Here's how the part is built. I have some questions about the finished solid (model axes, mm). Face numbers are marked on the shaded views. A direction names the side the tool comes from. Round coordinates to 2 decimals unless told otherwise and drop trailing zeros. Write each loop counter-clockwise with the first axis right and the second up, starting at its lowest first coordinate (ties: lowest second). Pieces come first, ordered by that corner, then holes. Notation, with made-up numbers: (33, 25) - (81, 25) arc R7 cw to (81, 37) - close; hole circle Ø11 at (6, 2.5). An arc over 180 degrees is marked (long way). One line per item, written item: value. Start each with the question number.
Item 1: Imagine slicing it at A-A, the plane y = 0. Please give me the cut outline in (x, z), then the cut area to 3 significant figures.
Item 2: If I drill on line 1 (Y direction, x = 20.75, z = -1.2); line 2 (Z direction, x = -2, y = -11.25); line 3 (X direction, y = 2.5, z = -10), over which ranges is the centre line in solid material (lowest first)?
Item 3: Imagine slicing it at B-B, the plane x = 20.75. Please give me the cut outline in (y, z), then the cut area to 3 significant figures.
Item 4: Imagine slicing it at D-D, the plane z = -9.5. Please give me the cut outline in (x, y).
Item 5: For P1, Ø3, axis at x = 21.5, z = -1.5, coming from the +Y side; P2, Ø6, axis at y = 5.5, z = -12.5, coming from the +X side; P3, Ø5, axis at x = 20.75, y = 0, coming from the -Z side; P4, Ø1.5, axis at x = -18.5, y = 9, coming from the -Z side, each with a flat end and sliding along its axis, tell me the tip position at first contact or that it passes through.
Item 6: Imagine slicing it at C-C, the plane x = 0. Please give me the cut outline in (y, z).
Item 7: For the marked faces 1 and 2, which set-ups out of +Z, -Z, +X, -X, +Y, -Y let a thin tool reach every point of the face, with its end or its side?
```python
from build123d import *

# Parameters (mm, degrees)
BOSS_EXTRUDE2_DEPTH = 2.6
SKETCH2_R           = 9
BOSS_EXTRUDE3_DEPTH = 16
REVOLVE1_ANGLE      = 180
SKETCH5_R           = 1.5
CUT_EXTRUDE1_DEPTH  = 16


with BuildPart() as part:
    # Sketch1 → Boss-Extrude2 (new body)
    with BuildSketch(Plane.XY):
        with BuildLine():
            Line((-26, -7.25), (-26, 7.25))
            Line((-26, 7.25), (-13.13, 7.25))
            ThreePointArc((-13.13, 7.25), (0, 14.998646606), (13.13, 7.25))
            Line((13.13, 7.25), (26, 7.25))
            Line((26, 7.25), (26, -7.25))
            Line((26, -7.25), (13.13, -7.25))
            ThreePointArc((13.13, -7.25), (0, -14.998646606), (-13.13, -7.25))
            Line((-13.13, -7.25), (-26, -7.25))
        make_face()
    extrude(amount=-BOSS_EXTRUDE2_DEPTH)

    # Sketch2 → Boss-Extrude3 (add)
    with BuildSketch(Plane.XY):
        Circle(SKETCH2_R)
    extrude(amount=-BOSS_EXTRUDE3_DEPTH)

    # Sketch3 → Revolve1 (revolve)
    with BuildSketch(Plane(origin=(0, 0, -16), x_dir=(-1, 0, 0), z_dir=(0, 0, -1))):
        with BuildLine():
            Line((-9, 0), (9, 0))
            ThreePointArc((9, 0), (0, 9), (-9, 0))
        make_face()
    revolve(axis=Axis((9, 0, -16), (-1, 0, 0)), revolution_arc=REVOLVE1_ANGLE)

    # Sketch5 → Cut-Extrude1 (cut)
    with BuildSketch(Plane.XY):
        with Locations((-20.75, 0)):
            Circle(SKETCH5_R)
        with Locations((20.75, 0)):
            Circle(SKETCH5_R)
    extrude(amount=-CUT_EXTRUDE1_DEPTH, mode=Mode.SUBTRACT)


solid = part.part
```
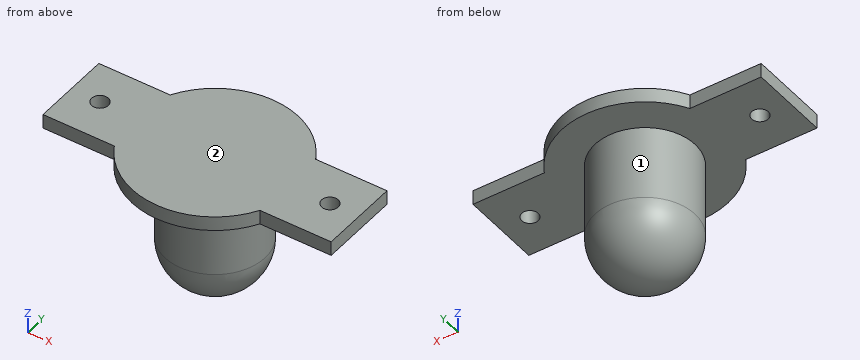
Values follow:
1. outline: (-26, -2.6) - (-22.25, -2.6) - (-22.25, 0) - (-26, 0) - close; (-19.25, -2.6) - (-9, -2.6) - (-9, -16) arc R9 ccw to (9, -16) - (9, -2.6) - (19.25, -2.6) - (19.25, 0) - (-19.25, 0) - close; (22.25, -2.6) - (26, -2.6) - (26, 0) - (22.25, 0) - close
1. area: 488 mm^2
2. line 1: y = -7.25 to -1.5, 1.5 to 7.25
2. line 2: z = -2.6 to 0
2. line 3: x = -8.65 to 8.65
3. outline: (-7.25, -2.6) - (-1.5, -2.6) - (-1.5, 0) - (-7.25, 0) - close; (1.5, -2.6) - (7.25, -2.6) - (7.25, 0) - (1.5, 0) - close
3. area: 29.9 mm^2
4. outline: circle Ø18 at (0, 0)
5. P1: stops at y = 7.25
5. P2: stops at x = 8.65
5. P3: stops at z = -2.6
5. P4: passes through
6. outline: (-15, -2.6) - (-9, -2.6) - (-9, -16) arc R9 ccw to (9, -16) - (9, -2.6) - (15, -2.6) - (15, 0) - (-15, 0) - close
7. face 1: -Z
7. face 2: +Z, +X, -X, +Y, -Y
